from build123d import *

# Parameters (mm, degrees)
SKETCH1_W                = 92
SKETCH1_H                = 77
SKETCH1_R                = 4
BOSS_EXTRUDE1_DEPTH      = 15
SKETCH1_3_R              = 4
BOSS_EXTRUDE2_DEPTH      = 15
BOSS_EXTRUDE2_DEPTH_BACK = 15
SKETCH2_R                = 3
CUT_EXTRUDE1_DEPTH       = 16
SKETCH2_3_W              = 11
SKETCH2_3_H              = 70
SKETCH2_3_W_2            = 10
CUT_EXTRUDE2_DEPTH       = 7


with BuildPart() as part:
    # Sketch1 → Boss-Extrude1 (new body)
    with BuildSketch(Plane.XY):
        with Locations((123.683888311, -870.843310138)):
            Rectangle(SKETCH1_W, SKETCH1_H)
        Polygon((169.683888311, -927.343310138), (217.683888311, -927.343310138), (217.683888311, -832.343310138), (169.683888311, -832.343310138), (169.683888311, -920.343310138), align=None)
        with Locations((207.683888311, -916.643310138)):
            Circle(SKETCH1_R, mode=Mode.SUBTRACT)
        Polygon((77.683888311, -909.343310138), (77.683888311, -920.343310138), (77.683888311, -927.343310138), (169.683888311, -927.343310138), (169.683888311, -920.343310138), (169.683888311, -909.343310138), align=None)
        with Locations((87.683888311, -916.643310138)):
            Circle(SKETCH1_R, mode=Mode.SUBTRACT)
        with Locations((159.683888311, -916.643310138)):
            Circle(SKETCH1_R, mode=Mode.SUBTRACT)
    extrude(amount=-BOSS_EXTRUDE1_DEPTH)

    # Sketch1_3 → Boss-Extrude2 (add, two sides)
    with BuildSketch(Plane.XY) as boss_extrude2_sk:
        with Locations((87.683888311, -916.643310138)):
            Circle(SKETCH1_3_R)
        with Locations((207.683888311, -916.643310138)):
            Circle(SKETCH1_3_R)
        with Locations((159.683888311, -916.643310138)):
            Circle(SKETCH1_3_R)
    extrude(amount=BOSS_EXTRUDE2_DEPTH)
    extrude(boss_extrude2_sk.sketch, amount=-BOSS_EXTRUDE2_DEPTH_BACK)

    # Sketch2 → Cut-Extrude1 (cut, through all)
    with BuildSketch(Plane.XY):
        with Locations((147.683888311, -887.343310138)):
            Circle(SKETCH2_R)
        with Locations((202.683888311, -887.343310138)):
            Circle(SKETCH2_R)
        with Locations((92.683888311, -887.343310138)):
            Circle(SKETCH2_R)
    extrude(amount=-CUT_EXTRUDE1_DEPTH, mode=Mode.SUBTRACT)

    # Sketch2_3 → Cut-Extrude2 (cut)
    with BuildSketch(Plane.XY):
        with Locations((103.683888311, -878.643310138)):
            Rectangle(SKETCH2_3_W, SKETCH2_3_H)
        with Locations((181.683888311, -878.643310138)):
            Rectangle(SKETCH2_3_W_2, SKETCH2_3_H)
    extrude(amount=-CUT_EXTRUDE2_DEPTH, mode=Mode.SUBTRACT)


solid = part.part
Could you check a few things on this model? Use its own coordinates, in mm. A direction names the side the tool comes from. Round coordinates to 2 decimals unless told otherwise and drop trailing zeros. Order: outer loops, then holes, each group sorted by start corner. A loop starts at its lowest first (then second) coordinate and runs counter-clockwise, first axis right, second up.
(1) Please list where these lines run through material, in increasing order: line 1 along X through (y, z) = (-845.5, -4.25); line 2 along Y through (x, z) = (179, -6.5); line 3 along Z through (x, y) = (102.5, -865).
Response values:
line 1: x = 77.68 to 98.18, 109.18 to 176.68, 186.68 to 217.68
line 2: y = -927.34 to -913.64, -843.64 to -832.34
line 3: z = -15 to -7
(2) Imagine slicing it at B-B (y = -894.5). Write out the boundary of the cut face in (x, z).
Response values:
outline: (77.68, -15) - (217.68, -15) - (217.68, 0) - (186.68, 0) - (186.68, -7) - (176.68, -7) - (176.68, 0) - (109.18, 0) - (109.18, -7) - (98.18, -7) - (98.18, 0) - (77.68, 0) - close
(3) Imagine slicing it at C-C (x = 202). Write out the boundary of the cut face in (y, z).
Response values:
outline: (-927.34, -15) - (-890.26, -15) - (-890.26, 0) - (-927.34, 0) - close; (-884.42, -15) - (-832.34, -15) - (-832.34, 0) - (-884.42, 0) - close
(4) Imagine slicing it at D-D (z = -5). Write out the boundary of the cut face in (x, y), plus the area to 3 significant figures.
Response values:
outline: (77.68, -927.34) - (217.68, -927.34) - (217.68, -832.34) - (77.68, -832.34) - close; hole circle Ø6 at (92.68, -887.34); hole (98.18, -913.64) - (109.18, -913.64) - (109.18, -843.64) - (98.18, -843.64) - close; hole circle Ø6 at (147.68, -887.34); hole (176.68, -913.64) - (186.68, -913.64) - (186.68, -843.64) - (176.68, -843.64) - close; hole circle Ø6 at (202.68, -887.34)
area: 11,700 mm2
(5) If we mould it in two halves opening along Y, with no side actions, what happens to faces 1 (the cylindrical face through (147.29, -884.37, -7.4)), 2 (the cylindrical face through (86.82, -920.55, 7.4)), 3 (the flat face through (217.684, -881, -7))? For each: released by +Y, released by -Y, zero draft, split by the parting line, or undercut.
Response values:
face 1: undercut
face 2: split by the parting line
face 3: zero draft
(6) Imagine slicing it at A-A (x = 185). Write out the boundary of the cut face in (y, z), plus the area to 3 significant figures.
Response values:
outline: (-927.34, -15) - (-832.34, -15) - (-832.34, 0) - (-843.64, 0) - (-843.64, -7) - (-913.64, -7) - (-913.64, 0) - (-927.34, 0) - close
area: 935 mm2
(7) Which directions (+Z, -Z, +X, -X, +Y, -Y) give clear straight access to the entire face, cutting with the end or side of a thin tool? Please do faces 4 (the flat face through (147, -879, -15)), 5 (the flat face through (182, -878, -7)).
Response values:
face 4: -Z, +X, -X, +Y, -Y
face 5: +Z
(8) I'm going to push flat-ended pins straight in: pin 1 (3.5 mm diameter, centred on x = 101.5, y = -882, fed in from +Z); pin 2 (4 mm diameter, centred on x = 164.5, z = 6.5, fed in from -Y); pin 3 (3.5 mm diameter, centred on x = 92.68, y = -887.34, fed in from -Z); pin 4 (2 mm diameter, centred on x = 151, y = -901.5, fed in from +Z). Where does each tip first touch, or does it pass through?
Response values:
pin 1: stops at z = -7
pin 2: stops at y = -919.48
pin 3: passes through
pin 4: stops at z = 0
